Check sheet for the modelled part. Datum: model origin and axes. Units: mm. A direction names the side the tool comes from. Give positions to 0.01 mm unless a question says otherwise; leave off trailing zeros. Loops run counter-clockwise (first coordinate to the right, second up) from the corner with the lowest first, then second, coordinate; pieces in that order, holes last. Notation, with made-up numbers: M -7.5,67 L 34.5,67 A14 ccw 34.5,84 Z; hole C 76.5,3.25 d9. An arc over 180 degrees is marked long. One line per question, with ' | ' between items. Start each with the question number.
from build123d import *

# Parameters (mm, degrees)
SALIENTE_EXTRUIR4_DEPTH = 14.2875
CROQUIS1_6_R            = 2.38125
SALIENTE_EXTRUIR5_DEPTH = 33.3375
CROQUIS1_7_R            = 2.38125
SALIENTE_EXTRUIR6_DEPTH = 39.6875


with BuildPart() as part:
    # Croquis1 → Saliente-Extruir4 (new body)
    with BuildSketch(Plane.XY):
        with BuildLine():
            Line((1.651, -8.567267885), (1.651, -8.152705854))
            Line((1.651, -8.152705854), (-1.524, -8.152705854))
            Line((-1.524, -8.152705854), (-1.524, -8.590768534))
            ThreePointArc((-1.524, -8.590768534), (-8.7249, 0), (-1.524, 8.590768534))
            Line((-1.524, 8.590768534), (-1.524, 8.152705854))
            Line((-1.524, 8.152705854), (1.651, 8.152705854))
            Line((1.651, 8.152705854), (1.651, 8.567267885))
            ThreePointArc((1.651, 8.567267885), (8.7249, 0), (1.651, -8.567267885))
        make_face()
        with BuildLine():
            ThreePointArc((3.77063, 2.921710837), (0, 4.77012), (-3.77063, 2.921710837))
            Line((-3.77063, 2.921710837), (-3.77063, -2.921710837))
            ThreePointArc((-3.77063, -2.921710837), (0, -4.77012), (3.77063, -2.921710837))
            Line((3.77063, -2.921710837), (3.77063, 2.921710837))
        make_face(mode=Mode.SUBTRACT)
    extrude(amount=SALIENTE_EXTRUIR4_DEPTH)

    # Croquis1_6 → Saliente-Extruir5 (add)
    with BuildSketch(Plane.XY):
        with BuildLine():
            Line((3.77063, -2.921710837), (3.77063, 2.921710837))
            ThreePointArc((3.77063, 2.921710837), (0, 4.77012), (-3.77063, 2.921710837))
            Line((-3.77063, 2.921710837), (-3.77063, -2.921710837))
            ThreePointArc((-3.77063, -2.921710837), (0, -4.77012), (3.77063, -2.921710837))
        make_face()
        Circle(CROQUIS1_6_R, mode=Mode.SUBTRACT)
    extrude(amount=SALIENTE_EXTRUIR5_DEPTH)

    # Croquis1_7 → Saliente-Extruir6 (add)
    with BuildSketch(Plane.XY):
        Circle(CROQUIS1_7_R)
    extrude(amount=SALIENTE_EXTRUIR6_DEPTH)


solid = part.part
Q1. Material ranges on probe 1 along Y at (x, z) = (-0.5, 3.5); probe 2 along Y at (x, z) = (0.25, 23); probe 3 along X at (y, z) = (2.75, 23), recorded low to high. Write a range as from..to.
Q2. Cross-section at D-D (x = 3). Record the cut outline in (y, z), and give its area (3 significant figures).
Q3. Cross-section at C-C (y = 0). Record the cut outline in (x, z).
Q4. Access from +Z, -Z, +X, -X, +Y, -Y to the whole of each face (thin tool, end or side, straight path). Record for faces 4 (the flat face through (0, -8.153, 7)), 5 (the cylindrical face through (-0.06, -4.77, 23.68)), 6 (the cylindrical face through (0.06, 4.77, 23.68)), 7 (the flat face through (4, 0, 14.288)).
Q5. Cross-section at B-B (z = 4). Record the cut outline in (x, y).
Q6. Cross-section at A-A (x = 0). Record the cut outline in (y, z).
Q7. Depth check by flat-ended pin: P1, Ø3, axis at y = 1, z = 23, coming from the -X side; P2, Ø3.5, axis at x = 0, z = 5.5, coming from the +Y side; P3, Ø4.5, axis at y = -1.5, z = 24, coming from the +X side; P4, Ø1, axis at x = 6.5, y = 5, coming from the +Z side. Enter the tip coordinate at first touch or a pass-through.
Q8. Draft check along X on faces 1 (the cylindrical face through (-1.89, -1.45, 36.47)), 2 (the flat face through (0, 8.153, 7)), 3 (the flat face through (-3.771, 0, 24)). Enter one of: released by +X, released by -X, zero draft, split by the parting line, or undercut.
Solved:
1) probe 1: y = -8.15..8.15 | probe 2: y = -4.76..4.76 | probe 3: x = -3.77..3.77
2) outline: M -8.19,0 L 8.19,0 L 8.19,14.29 L 3.71,14.29 L 3.71,33.34 L -3.71,33.34 L -3.71,14.29 L -8.19,14.29 Z | area: 375 mm²
3) outline: M -8.72,0 L 8.72,0 L 8.72,14.29 L 3.77,14.29 L 3.77,33.34 L 2.38,33.34 L 2.38,39.69 L -2.38,39.69 L -2.38,33.34 L -3.77,33.34 L -3.77,14.29 L -8.72,14.29 Z
4) face 4: +Z, -Z, -Y | face 5: +Z, -Y | face 6: +Z, +Y | face 7: +Z
5) outline: M -1.52,-8.59 L -1.52,-8.15 L 1.65,-8.15 L 1.65,-8.57 A8.72 ccw 1.65,8.57 L 1.65,8.15 L -1.52,8.15 L -1.52,8.59 A8.72 ccw Z
6) outline: M -8.15,0 L 8.15,0 L 8.15,14.29 L 4.77,14.29 L 4.77,33.34 L 2.38,33.34 L 2.38,39.69 L -2.38,39.69 L -2.38,33.34 L -4.77,33.34 L -4.77,14.29 L -8.15,14.29 Z
7) P1: stops at x = -3.77 | P2: stops at y = 8.59 | P3: stops at x = 3.77 | P4: stops at z = 14.29
8) face 1: split by the parting line | face 2: undercut | face 3: released by -X
